Can you work these out from the drawing? Everything is in mm from the part's minimum corner. A direction names the side the tool comes from. Coordinates: 2 decimals unless noted, no trailing zeros. Loops run counter-clockwise (first coordinate to the right, second up) from the corner with the lowest first, then second, coordinate; pieces in that order, holes last.
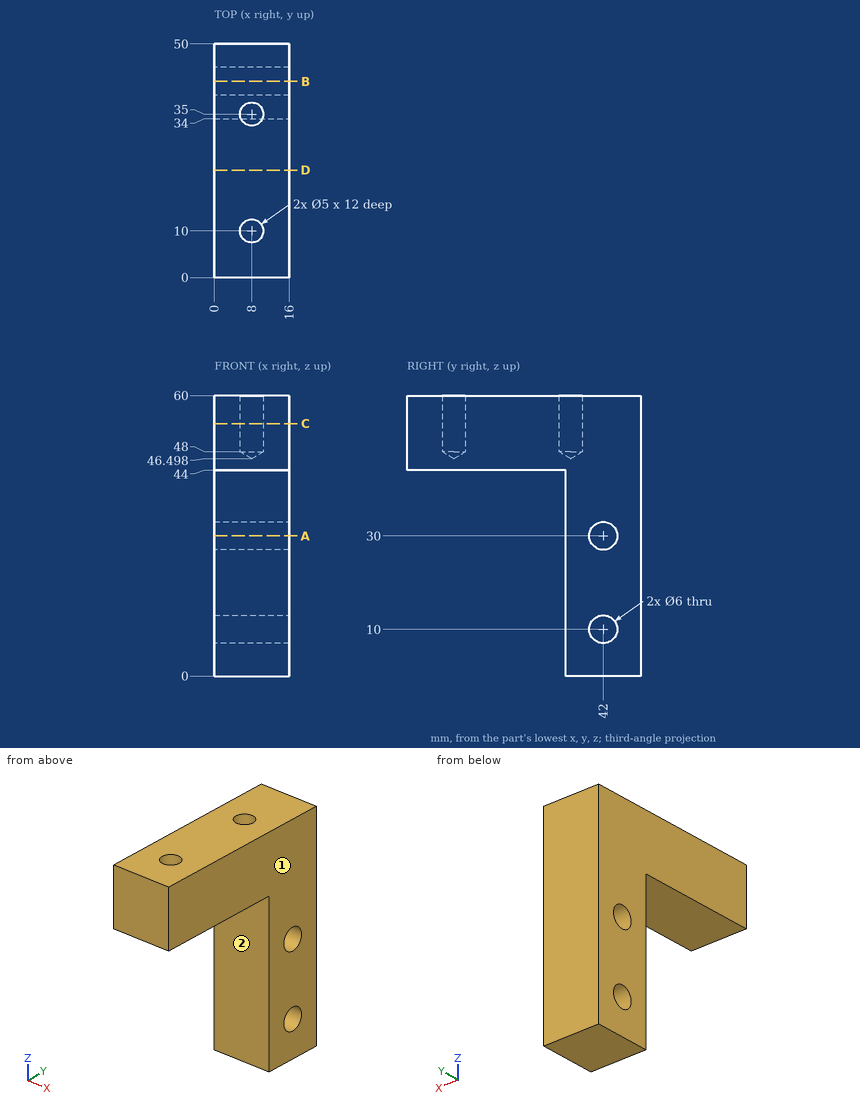
(1) Which directions (+Z, -Z, +X, -X, +Y, -Y) give clear straight access to the entire face, cutting with the end or side of a thin tool? Please do the marked faces 1 and 2.
Answers:
face 1: +Z, -Z, +X, +Y, -Y
face 2: -Z, +X, -X, -Y
(2) For pin 1 (5 mm diameter, centred on x = 11.5, y = 18, fed in from -Z); pin 2 (1.5 mm diameter, centred on x = 8.5, z = 10.5, fed in from -Y); pin 3 (3 mm diameter, centred on x = 8, y = 35, fed in from +Z), each with a flat end and sliding along its axis, tell me the tip position at first contact or that it passes through.
Answers:
pin 1: stops at z = 44
pin 2: stops at y = 34
pin 3: stops at z = 47.4
(3) Imagine slicing it at A-A, the plane z = 30. Write out the boundary of the cut face in (x, y).
Answers:
outline: (0, 34) - (16, 34) - (16, 39) - (0, 39) - close; (0, 45) - (16, 45) - (16, 50) - (0, 50) - close
(4) Imagine slicing it at D-D, the plane y = 23. Write out the boundary of the cut face in (x, z), and give its area (3 significant figures).
Answers:
outline: (0, 44) - (16, 44) - (16, 60) - (0, 60) - close
area: 256 mm2
(5) Imagine slicing it at B-B, the plane y = 42. Write out the boundary of the cut face in (x, z), and give its area (3 significant figures).
Answers:
outline: (0, 0) - (16, 0) - (16, 7) - (0, 7) - close; (0, 13) - (16, 13) - (16, 27) - (0, 27) - close; (0, 33) - (16, 33) - (16, 60) - (0, 60) - close
area: 768 mm2
(6) Imagine slicing it at C-C, the plane z = 54. Write out the boundary of the cut face in (x, y).
Answers:
outline: (0, 0) - (16, 0) - (16, 50) - (0, 50) - close; hole circle Ø5 at (8, 10); hole circle Ø5 at (8, 35)
(7) I need wall thicknesses on probe 1 along Y at (x, z) = (8, 56.5); probe 2 along X at (y, z) = (10, 55); probe 3 along Y at (x, z) = (6.25, 10). Which ranges of each line are inside material? Lowest first, please.
Answers:
probe 1: y = 0 to 7.5, 12.5 to 32.5, 37.5 to 50
probe 2: x = 0 to 5.5, 10.5 to 16
probe 3: y = 34 to 39, 45 to 50
